from build123d import *

# Parameters (mm, degrees)
SKETCH_1_W          = 60
SKETCH_1_H          = 30
EXTRUDE_1_DEPTH     = 2
SKETCH_2_W          = 3
SKETCH_2_H          = 3
EXTRUDE_2_DEPTH     = 1
EXTRUDE_START       = -4
EXTRUDE_3_DEPTH     = 5
CUT_EXTRUDE_1_REACH = 60.969
FILLET_1_R          = 0.1
FILLET_2_R          = 0.2


with BuildPart() as part:
    # Sketch 1 → Extrude 1 (new body)
    with BuildSketch(Plane.XY):
        with Locations((0, 7.5)):
            Rectangle(SKETCH_1_W, SKETCH_1_H)
    extrude(amount=-EXTRUDE_1_DEPTH)

    # Sketch 2 → Extrude 2 (add)
    with BuildSketch(Plane.XY):
        with Locations((-22.5, 0)):
            Rectangle(SKETCH_2_W, SKETCH_2_H)
    extrude_2 = extrude(amount=EXTRUDE_2_DEPTH)

    # Sketch 3 → Extrude 3 (add)
    with BuildSketch(Plane.XZ.offset(1.5).offset(EXTRUDE_START)):
        with BuildLine():
            Line((-24.45, 2.5), (-20.55, 2.5))
            Line((-20.55, 2.5), (-20.55, 1.555590279))
            ThreePointArc((-20.55, 1.555590279), (-20.719957697, 1.088161527), (-21, 0.677124344))
            Line((-21, 0.677124344), (-24, 0.677124344))
            ThreePointArc((-24, 0.677124344), (-24.280042303, 1.088161527), (-24.45, 1.555590279))
            Line((-24.45, 1.555590279), (-24.45, 2.5))
        make_face()
    extrude_3 = extrude(amount=EXTRUDE_3_DEPTH)

    # Sketch 4 → Cut-Extrude 1 (cut, up to next)
    with BuildSketch(Plane.ZY.offset(24.45), mode=Mode.PRIVATE) as cut_extrude_1_sk1:
        with BuildLine():
            Line((2.5, 1.95), (1.555590279, 1.95))
            ThreePointArc((1.555590279, 1.95), (1.088161527, 1.780042303), (0.677124344, 1.5))
            Line((0.677124344, 1.5), (0.677124344, 2.5))
            Line((0.677124344, 2.5), (2.5, 2.5))
            Line((2.5, 2.5), (2.5, 1.95))
        make_face()
    cut_extrude_1_tool1 = extrude(cut_extrude_1_sk1.sketch, amount=-CUT_EXTRUDE_1_REACH, mode=Mode.PRIVATE) & part.part
    # Sketch 4 → Cut-Extrude 1 (cut, up to next)
    with BuildSketch(Plane.ZY.offset(24.45), mode=Mode.PRIVATE) as cut_extrude_1_sk2:
        with BuildLine():
            Line((0.677124344, -2.5), (2.5, -2.5))
            Line((2.5, -2.5), (2.5, -1.95))
            Line((2.5, -1.95), (1.555590279, -1.95))
            ThreePointArc((1.555590279, -1.95), (1.088161527, -1.780042303), (0.677124344, -1.5))
            Line((0.677124344, -1.5), (0.677124344, -2.5))
        make_face()
    cut_extrude_1_tool2 = extrude(cut_extrude_1_sk2.sketch, amount=-CUT_EXTRUDE_1_REACH, mode=Mode.PRIVATE) & part.part
    cut_extrude_1_1 = cut_extrude_1_tool1.solids().sort_by_distance((-24.45, 2.169375, 1.500125))[0]
    add(cut_extrude_1_1, mode=Mode.SUBTRACT)
    cut_extrude_1_2 = cut_extrude_1_tool2.solids().sort_by_distance((-24.45, -2.169375, 1.500125))[0]
    add(cut_extrude_1_2, mode=Mode.SUBTRACT)
    cut_extrude_1 = cut_extrude_1_1 + cut_extrude_1_2  # Cut-Extrude 1 as one shape, for the pattern or mirror that repeats it

    # Mirror 1: Extrude 2, Extrude 3, Cut-Extrude 1 across plane
    add(extrude_2.mirror(Plane(origin=(0, 0, 0), x_dir=(0, 0, 1), z_dir=(1, 0, 0))))
    add(extrude_3.mirror(Plane(origin=(0, 0, 0), x_dir=(0, 0, 1), z_dir=(1, 0, 0))))
    add(cut_extrude_1.mirror(Plane(origin=(0, 0, 0), x_dir=(0, 0, 1), z_dir=(1, 0, 0))), mode=Mode.SUBTRACT)

    # Fillet 1
    fillet_1_edges = [part.edges().sort_by_distance(p)[0] for p in [
        (22.5, -1.95, 2.5),
        (24.45, 0, 2.5),
        (20.55, 0, 2.5),
        (22.5, 1.95, 2.5),
        (-22.5, -1.95, 2.5),
        (-20.55, 0, 2.5),
        (-24.45, 0, 2.5),
        (-22.5, 1.95, 2.5),
    ]]
    fillet(fillet_1_edges, radius=FILLET_1_R)

    # Fillet 2
    fillet_2_edges = [part.edges().sort_by_distance(p)[0] for p in [
        (30, 7.5, -2),
        (0, 22.5, -2),
        (-30, 7.5, -2),
        (0, 22.5, 0),
        (30, 7.5, 0),
        (0, -7.5, 0),
        (-30, 7.5, 0),
        (0, -7.5, -2),
        (-30, 22.5, -1),
        (30, 22.5, -1),
        (30, -7.5, -1),
        (-30, -7.5, -1),
    ]]
    fillet(fillet_2_edges, radius=FILLET_2_R)


solid = part.part
The model under review builds one solid part; all positions refer to its coordinate system, in mm. Coordinates: 2 decimals unless noted, no trailing zeros. Write each loop counter-clockwise with the first axis right and the second up, starting at its lowest first coordinate (ties: lowest second). Pieces come first, ordered by that corner, then holes. Notation, with made-up numbers: (-40, -33.5) -> (-32, -33.5) arc R31 cw to (-32, -9.5) -> close; hole circle Ø4 at (71, 18.5). An arc over 180 degrees is marked (long way). Answer in a Markdown table with one row per item.
1. We need section C-C, the plane y = 18.5. State the section outline as (x, z) points, and give its area (3 significant figures).
Answers below:
| item | result |
|---|---|
| outline | (-30, -1.8) arc R0.2 ccw to (-29.8, -2) -> (29.8, -2) arc R0.2 ccw to (30, -1.8) -> (30, -0.2) arc R0.2 ccw to (29.8, 0) -> (-29.8, 0) arc R0.2 ccw to (-30, -0.2) -> close |
| area | 120 mm^2 |
2. Clearance check with flat-ended pins moving along their axes: pin 1 Ø0.7 at (x, z) = (-22.5, 0.5) entering from -Y; pin 2 Ø0.5 at (y, z) = (-0.5, 0.5) entering from +X; pin 3 Ø0.7 at (x, z) = (-23.5, 2) entering from +Y; pin 4 Ø1 at (x, z) = (18.5, 1) entering from -Y. State where each tip first meets the part, or that it passes through.
Answers below:
| item | result |
|---|---|
| pin 1 | stops at y = -1.64 |
| pin 2 | stops at x = 24.06 |
| pin 3 | stops at y = 1.95 |
| pin 4 | passes through |
3. We need section B-B, the plane x = -13. State the section outline as (y, z) points.
Answers below:
| item | result |
|---|---|
| outline | (-7.5, -1.8) arc R0.2 ccw to (-7.3, -2) -> (22.3, -2) arc R0.2 ccw to (22.5, -1.8) -> (22.5, -0.2) arc R0.2 ccw to (22.3, 0) -> (-7.3, 0) arc R0.2 ccw to (-7.5, -0.2) -> close |
4. Wall thickness on probe 1 along X at (y, z) = (-1.5, 1.8); probe 2 along Z at (x, y) = (-26.5, 12); probe 3 along X at (y, z) = (0, 0.7): over which ranges is each line inside the solid? List them lowest first. Write a range as [from, to].
Answers below:
| item | result |
|---|---|
| probe 1 | x = [-24.45, -20.55], [20.55, 24.45] |
| probe 2 | z = [-2, 0] |
| probe 3 | x = [-24.02, -20.98], [20.98, 24.02] |
5. We need section A-A, the plane y = -0.25. State the section outline as (x, z) points, and give its area (3 significant figures).
Answers below:
| item | result |
|---|---|
| outline | (-30, -1.8) arc R0.2 ccw to (-29.8, -2) -> (29.8, -2) arc R0.2 ccw to (30, -1.8) -> (30, -0.2) arc R0.2 ccw to (29.8, 0) -> (24, 0) -> (24, 0.68) arc R2 ccw to (24.45, 1.56) -> (24.45, 2.4) arc R0.1 ccw to (24.35, 2.5) -> (20.65, 2.5) arc R0.1 ccw to (20.55, 2.4) -> (20.55, 1.56) arc R2 ccw to (21, 0.68) -> (21, 0) -> (-21, 0) -> (-21, 0.68) arc R2 ccw to (-20.55, 1.56) -> (-20.55, 2.4) arc R0.1 ccw to (-20.65, 2.5) -> (-24.35, 2.5) arc R0.1 ccw to (-24.45, 2.4) -> (-24.45, 1.56) arc R2 ccw to (-24, 0.68) -> (-24, 0) -> (-29.8, 0) arc R0.2 ccw to (-30, -0.2) -> close |
| area | 138 mm^2 |
6. Draft analysis for pull direction X (two halves, no side actions). For faces 1 (the flat face through (0, -7.5, -1)), 2 (the flat face through (30, 7, -1)), 3 (the flat face through (-30, 7, -1)), state which applies: +X half, -X half, draft (parallel to the pull), parting line (faces both ways), or undercut.
Answers below:
| item | result |
|---|---|
| face 1 | draft |
| face 2 | +X half |
| face 3 | -X half |
